Geometry: final body of the model. Coordinates: model frame, mm. Give positions to 0.01 mm unless a question says otherwise; leave off trailing zeros. Order: outer loops, then holes, each group sorted by start corner. A loop starts at its lowest first (then second) coordinate and runs counter-clockwise, first axis right, second up. Notation, with made-up numbers: (56.5, 67.25) -> (80.5, 67.25) arc R23 ccw to (80.5, 104.25) -> close; hole circle Ø1 at (-16.5, 10). An arc over 180 degrees is marked (long way). One line per item, written item: value. Start each with the question number.
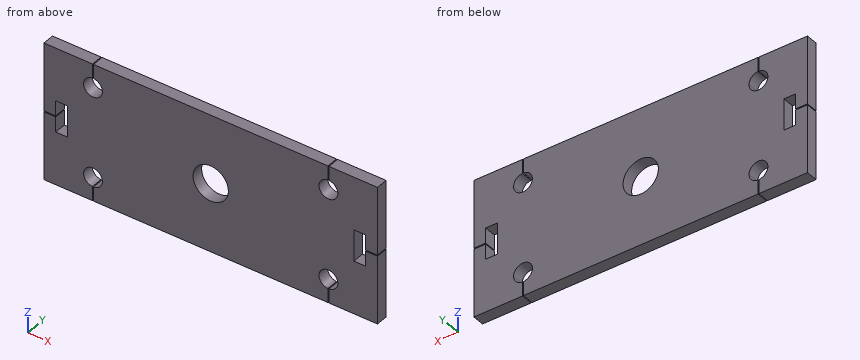
```python
from build123d import *

# Parameters (mm, degrees)
ESBO_O2_W                = 85
ESBO_O2_H                = 35
RESSALTO_EXTRUS_O2_DEPTH = 3
ESBO_O3_W                = 3.01
ESBO_O3_H                = 8.005
CORTE_EXTRUS_O1_DEPTH    = 47.059743812
FURO_COM_FOLGA_DE_M41_D  = 4.8
FURO_COM_FOLGA_DE_M81_D  = 9
ESBO_O13_W               = 0.25
ESBO_O13_H               = 3.603257419
ESBO_O13_W_2             = 3
ESBO_O13_H_2             = 0.25
CORTE_EXTRUS_O2_DEPTH    = 47.059743812


with BuildPart() as part:
    # Esboço2 → Ressalto-extrusão2 (new body)
    with BuildSketch(Plane(origin=(0, 0, 0), x_dir=(1, 0, 0), z_dir=(0, 1, 0))):
        Rectangle(ESBO_O2_W, ESBO_O2_H)
    extrude(amount=RESSALTO_EXTRUS_O2_DEPTH)

    # Esboço3 → Corte-extrusão1 (cut, through all)
    with BuildSketch(Plane.XZ):
        with Locations((-37.995, 0)):
            Rectangle(ESBO_O3_W, ESBO_O3_H)
        with Locations((37.995, 0)):
            Rectangle(ESBO_O3_W, ESBO_O3_H)
    extrude(amount=-CORTE_EXTRUS_O1_DEPTH, mode=Mode.SUBTRACT)

    # Furo com folga de M41 (through all)
    with Locations(Plane(origin=(0, 0, 0), x_dir=(-1, 0, 0), z_dir=(0, -1, 0))):
        with Locations((30, -11.5), (30, 11.5), (-30, 11.5), (-30, -11.5)):
            Hole(FURO_COM_FOLGA_DE_M41_D / 2)

    # Furo com folga de M81 (through all)
    with Locations(Plane(origin=(0, 3, 0), x_dir=(1, 0, 0), z_dir=(0, 1, 0))):
        with Locations((0, 0)):
            Hole(FURO_COM_FOLGA_DE_M81_D / 2)

    # Esboço13 → Corte-extrusão2 (cut, through all)
    with BuildSketch(Plane(origin=(0, 3, 0), x_dir=(1, 0, 0), z_dir=(0, 1, 0))):
        with Locations((-30, 15.698371291)):
            Rectangle(ESBO_O13_W, ESBO_O13_H)
        with Locations((-41, 0)):
            Rectangle(ESBO_O13_W_2, ESBO_O13_H_2)
        with Locations((-30, -15.698371291)):
            Rectangle(ESBO_O13_W, ESBO_O13_H)
        with Locations((30, -15.698371291)):
            Rectangle(ESBO_O13_W, ESBO_O13_H)
        with Locations((41, 0)):
            Rectangle(ESBO_O13_W_2, ESBO_O13_H_2)
        with Locations((30, 15.698371291)):
            Rectangle(ESBO_O13_W, ESBO_O13_H)
    extrude(amount=-CORTE_EXTRUS_O2_DEPTH, mode=Mode.SUBTRACT)


solid = part.part
```
1. Cut plane B-B, the plane z = -13. Return loops of the section in (x, y).
2. Cut plane A-A, the plane x = 0. Return loops of the section in (y, z), then the cut area to 3 significant figures.
3. Material intervals for L1, parallel to X at y = 2.15, z = 11.5; L2, parallel to X at y = 1.55, z = -10; L3, parallel to Z at x = 2, y = 2.1, sorted ascending. Write a range as [from, to].
4. Pin query (flat end, axial travel): P1, Ø10, axis at x = -4.5, z = -6, coming from the -Y side. Return the tip coordinate at first contact, or that it passes through.
Answers follow:
1. outline: (-42.5, 0) -> (-31.87, 0) -> (-31.87, 3) -> (-42.5, 3) -> close; (-28.13, 0) -> (28.13, 0) -> (28.13, 3) -> (-28.13, 3) -> close; (31.87, 0) -> (42.5, 0) -> (42.5, 3) -> (31.87, 3) -> close
2. outline: (0, -17.5) -> (3, -17.5) -> (3, -4.5) -> (0, -4.5) -> close; (0, 4.5) -> (3, 4.5) -> (3, 17.5) -> (0, 17.5) -> close
2. area: 78.0 mm²
3. L1: x = [-42.5, -32.4], [-27.6, 27.6], [32.4, 42.5]
3. L2: x = [-42.5, -31.87], [-28.13, 28.13], [31.87, 42.5]
3. L3: z = [-17.5, -4.03], [4.03, 17.5]
4. P1: stops at y = 0
